Model file for the job. Use its own axes, mm. Round coordinates to 2 decimals unless told otherwise and drop trailing zeros. Write each loop counter-clockwise with the first axis right and the second up, starting at its lowest first coordinate (ties: lowest second). Pieces come first, ordered by that corner, then holes. Notation, with made-up numbers: (5.25, 43) - (58.25, 43) arc R23 ccw to (58.25, 73) - close; hole circle Ø1 at (77.5, -20.5). An arc over 180 degrees is marked (long way). One line per item, written item: value.
from build123d import *

# Parameters (mm, degrees)
BOSS_EXTRUDE1_DEPTH = 198
CUT_EXTRUDE3_DEPTH  = 206.200438596
BOSS_EXTRUDE2_DEPTH = 1.636319424
FILLET1_R           = 1


with BuildPart() as part:
    # Sketch1 → Boss-Extrude1 (new body)
    with BuildSketch(Plane.XY):
        with BuildLine():
            Line((2.54, 0), (35.56, 0))
            ThreePointArc((35.56, 0), (37.356051224, -0.743948776), (38.1, -2.54))
            Line((38.1, -2.54), (38.1, -35.56))
            ThreePointArc((38.1, -35.56), (37.356051224, -37.356051224), (35.56, -38.1))
            Line((35.56, -38.1), (2.54, -38.1))
            ThreePointArc((2.54, -38.1), (0.743948776, -37.356051224), (0, -35.56))
            Line((0, -35.56), (0, -2.54))
            ThreePointArc((0, -2.54), (0.743948776, -0.743948776), (2.54, 0))
        make_face()
        with BuildLine():
            Line((5.3086, -2.7686), (32.7914, -2.7686))
            ThreePointArc((32.7914, -2.7686), (34.587451224, -3.512548776), (35.3314, -5.3086))
            Line((35.3314, -5.3086), (35.3314, -32.7914))
            ThreePointArc((35.3314, -32.7914), (34.587451224, -34.587451224), (32.7914, -35.3314))
            Line((32.7914, -35.3314), (5.3086, -35.3314))
            ThreePointArc((5.3086, -35.3314), (3.512548776, -34.587451224), (2.7686, -32.7914))
            Line((2.7686, -32.7914), (2.7686, -5.3086))
            ThreePointArc((2.7686, -5.3086), (3.512548776, -3.512548776), (5.3086, -2.7686))
        make_face(mode=Mode.SUBTRACT)
    extrude(amount=BOSS_EXTRUDE1_DEPTH)

    # Sketch3 → Cut-Extrude3 (cut, through all)
    with BuildSketch(Plane(origin=(38.1, 0, 0), x_dir=(0, 0, -1), z_dir=(1, 0, 0))):
        Polygon((-198, 0), (-194.66668192, -38.1), (-198, -38.1), align=None)
    extrude(amount=-CUT_EXTRUDE3_DEPTH, mode=Mode.SUBTRACT)

    # Sketch4 → Boss-Extrude2 (add)
    with BuildSketch(Plane(origin=(0, -17.191169589, 196.495967548), x_dir=(1, 0, 0), z_dir=(0, -0.08715574274765185, 0.9961946980917462))):
        with BuildLine():
            Line((2.54, -20.988698746), (35.56, -20.988698746))
            add(Edge.make_bspline(
                [(35.56, -20.988698746), (38.1, -20.988698746), (38.1, -18.438996359)],
                knots=[0, 0, 0, 1.570796327, 1.570796327, 1.570796327], degree=2, weights=[1, 0.707106781, 1]))
            Line((38.1, -18.438996359), (38.1, 14.707134677))
            add(Edge.make_bspline(
                [(38.1, 14.707134677), (38.1, 17.256837064), (35.56, 17.256837064)],
                knots=[4.71238898, 4.71238898, 4.71238898, 6.283185307, 6.283185307, 6.283185307], degree=2, weights=[1, 0.707106781, 1]))
            Line((35.56, 17.256837064), (2.54, 17.256837064))
            add(Edge.make_bspline(
                [(2.54, 17.256837064), (0, 17.256837064), (0, 14.707134677)],
                knots=[3.141592654, 3.141592654, 3.141592654, 4.71238898, 4.71238898, 4.71238898], degree=2, weights=[1, 0.707106781, 1]))
            Line((0, 14.707134677), (0, -18.438996359))
            add(Edge.make_bspline(
                [(0, -18.438996359), (0, -20.988698746), (2.54, -20.988698746)],
                knots=[4.71238898, 4.71238898, 4.71238898, 6.283185307, 6.283185307, 6.283185307], degree=2, weights=[1, 0.707106781, 1]))
        make_face()
        with BuildLine():
            Line((35.3314, 11.927959074), (35.3314, -15.659820757))
            add(Edge.make_bspline(
                [(32.7914, -18.209523144), (35.3314, -18.209523144), (35.3314, -15.659820757)],
                knots=[0, 0, 0, 1.570796327, 1.570796327, 1.570796327], degree=2, weights=[1, 0.707106781, 1]))
            Line((32.7914, -18.209523144), (5.3086, -18.209523144))
            add(Edge.make_bspline(
                [(2.7686, -15.659820757), (2.7686, -18.209523144), (5.3086, -18.209523144)],
                knots=[4.71238898, 4.71238898, 4.71238898, 6.283185307, 6.283185307, 6.283185307], degree=2, weights=[1, 0.707106781, 1]))
            Line((2.7686, -15.659820757), (2.7686, 11.927959074))
            add(Edge.make_bspline(
                [(5.3086, 14.477661462), (2.7686, 14.477661462), (2.7686, 11.927959074)],
                knots=[3.141592654, 3.141592654, 3.141592654, 4.71238898, 4.71238898, 4.71238898], degree=2, weights=[1, 0.707106781, 1]))
            Line((5.3086, 14.477661462), (32.7914, 14.477661462))
            add(Edge.make_bspline(
                [(35.3314, 11.927959074), (35.3314, 14.477661462), (32.7914, 14.477661462)],
                knots=[1.570796327, 1.570796327, 1.570796327, 3.141592654, 3.141592654, 3.141592654], degree=2, weights=[1, 0.707106781, 1]))
        make_face(mode=Mode.SUBTRACT)
    extrude(amount=BOSS_EXTRUDE2_DEPTH)

    # Fillet1
    fillet1_edges = [part.edges().sort_by_distance(p)[0] for p in [
        (35.3314, -19.192614635, 197.963433694),
        (34.589162497, -34.728352955, 196.604232712),
        (19.05, -35.474014635, 196.538995768),
        (3.510837922, -34.728353374, 196.604232675),
        (2.7686, -19.192614635, 197.963433694),
        (3.510837503, -3.656876315, 199.322634677),
        (19.05, -2.911214635, 199.387871621),
        (34.589162078, -3.656875896, 199.322634714),
        (0, -19.192614635, 197.963433694),
        (0.742237922, -37.496953374, 196.362011561),
        (19.05, -38.242614635, 196.296774654),
        (37.357762497, -37.496952955, 196.362011598),
        (38.1, -19.192614635, 197.963433694),
        (37.357762078, -0.888275896, 199.564855827),
        (19.05, -0.142614635, 199.630092735),
        (0.742237503, -0.888276315, 199.564855791),
    ]]
    fillet(fillet1_edges, radius=FILLET1_R)


solid = part.part
1. Wall check: probe 1 along Y at (x, z) = (27.5, 119); probe 2 along X at (y, z) = (-10.5, 97.5); probe 3 along Y at (x, z) = (35.5, 131). Give the ranges that are in metal, low to high. Write a range as [from, to].
Report:
probe 1: [-38.1, -35.33], [-2.77, 0]
probe 2: [0, 2.77], [35.33, 38.1]
probe 3: [-38.1, 0]
2. Drop flat-ended pins along their axis: pin 1 (22 mm diameter, centred on x = 22, z = 80.5, fed in from -Y); pin 2 (12 mm diameter, centred on x = 8.5, y = -20, fed in from +Z); pin 3 (8 mm diameter, centred on x = 34, y = -14, fed in from -Z). Give the stop position or say it passes through.
Report:
pin 1: y = -38.1
pin 2: z = 197.59
pin 3: z = 0
3. Mould opens along Y. For faces 1 (the face through (37.8, -18.9, 197.7)), 2 (the face through (19, -35.331, 96)), 3 (the face through (35.331, -19, 97)), 4 (the face through (0, -18, 96)) say: released by +Y, released by -Y, zero draft, split by the parting line, or undercut.
Report:
face 1: released by -Y
face 2: undercut
face 3: undercut
face 4: zero draft
4. Band-saw the part on A-A on z = 158. Write the cut outline in (x, y), plus the area to 3 significant figures.
Report:
outline: (0, -35.56) arc R2.54 ccw to (2.54, -38.1) - (35.56, -38.1) arc R2.54 ccw to (38.1, -35.56) - (38.1, -2.54) arc R2.54 ccw to (35.56, 0) - (2.54, 0) arc R2.54 ccw to (0, -2.54) - close; hole (2.77, -32.79) arc R2.54 ccw to (5.31, -35.33) - (32.79, -35.33) arc R2.54 ccw to (35.33, -32.79) - (35.33, -5.31) arc R2.54 ccw to (32.79, -2.77) - (5.31, -2.77) arc R2.54 ccw to (2.77, -5.31) - close
area: 391 mm²
5. Band-saw the part on B-B on x = 30.5. Write the cut outline in (y, z), plus the area to 3 significant figures.
Report:
outline: (-38.16, 195.3) - (-38.1, 194.67) - (-38.1, 0) - (-35.33, 0) - (-35.33, 194.91) - (-35.39, 195.54) arc R1 ccw to (-36.47, 196.45) - (-37.25, 196.38) arc R1 ccw to start; (-2.82, 198.39) - (-2.77, 197.76) - (-2.77, 0) - (0, 0) - (0, 198) - (-0.06, 198.63) arc R1 ccw to (-1.14, 199.54) - (-1.92, 199.48) arc R1 ccw to start
area: 1,100 mm²
